```python
from build123d import *

# Parameters (mm, degrees)
F0_W          = 64
F0_H          = 73
F1_DEPTH      = 5.5
F2_DEPTH      = 15.5
F3_W          = 15
F3_H          = 0.5
F4_DEPTH      = 3
F6_W          = 2.5
F6_H          = 15
F7_DEPTH      = 5.501
F8_SIZE       = 2.5
F9_R          = 1.5
F10_R         = 7.5
F11_T1_DEPTH  = 58
F11_T3_DEPTH  = 49
F11_T5_DEPTH  = 2.5
F11_T7_DEPTH  = 15
F11_T10_ANGLE = 90
F11_T12_ANGLE = 90
F11_T14_ANGLE = 90
F11_T16_ANGLE = 90
F11_T21_DEPTH = 5.0870857546
F11_T25_DEPTH = 17.5870857546
F11_T32_DEPTH = 5.0870857546
F11_T36_DEPTH = 17.5870857546
F11_T43_DEPTH = 17.5870857546
F11_T47_DEPTH = 5.0870857546
F11_T54_DEPTH = 5.0870857546
F11_T58_DEPTH = 17.5870857546
F12_SIZE2     = 0.5773502692
F12_SIZE      = 1


# Not quite as in the source:
# - a fillet or chamfer that OpenCascade refuses, or shapes differently, is made with other operations: its cross-section is extruded or revolved along the edge and cut away or added


with BuildPart() as f1:
    # F0 (on Top) → F1 (new body)
    with BuildSketch(Plane.XY):
        Rectangle(F0_W, F0_H)
        Polygon((-22.5, 7.5), (-22.5, 30), (22.5, 30), (22.5, 7.5), (25.5, 7.5), (25.5, -7.5), (22.5, -7.5), (22.5, -30), (-22.5, -30), (-22.5, -7.5), (-25.5, -7.5), (-25.5, 7.5), align=None, mode=Mode.SUBTRACT)
        Polygon((22.5, 30), (-22.5, 30), (-22.5, 7.5), (-25.5, 7.5), (-25.5, -7.5), (-22.5, -7.5), (-22.5, -30), (22.5, -30), (22.5, -7.5), (25.5, -7.5), (25.5, 7.5), (22.5, 7.5), align=None)
    extrude(amount=-F1_DEPTH)

    # F0 (on Top) → F2 (join)
    with BuildSketch(Plane.XY):
        Rectangle(F0_W, F0_H)
        Polygon((-22.5, 7.5), (-22.5, 30), (22.5, 30), (22.5, 7.5), (25.5, 7.5), (25.5, -7.5), (22.5, -7.5), (22.5, -30), (-22.5, -30), (-22.5, -7.5), (-25.5, -7.5), (-25.5, 7.5), align=None, mode=Mode.SUBTRACT)
    extrude(amount=F2_DEPTH)

    # F3 (on face) → F4 (join, through all)
    with BuildSketch(Plane.YZ.offset(-25.5)):
        with Locations((0, 15.25)):
            Rectangle(F3_W, F3_H)
    extrude(amount=F4_DEPTH)

    # F5: F1 across plane


with BuildPart() as f1_1:
    add(f1.part)
    add(f1.part.mirror(Plane.YZ))

    # F6 (on face) → F7 (cut, through all)
    with BuildSketch(Plane.XY):
        with Locations((-17.75, 20.5)):
            Rectangle(F6_W, F6_H)
    extrude(amount=-F7_DEPTH, mode=Mode.SUBTRACT)

    # F8
    f8_edges = [f1_1.edges().sort_by_distance(p)[0] for p in [
        (-22.5, -7.5, 7.5),
        (-22.5, 7.5, 7.5),
        (22.5, 7.5, 7.5),
        (22.5, -7.5, 7.5),
    ]]
    chamfer(f8_edges, length=F8_SIZE)

    # F9
    f9_edges = [f1_1.edges().sort_by_distance(p)[0] for p in [
        (-22.5, 30, 7.75),
        (-22.5, -30, 7.75),
        (22.5, 30, 7.75),
        (22.5, -30, 7.75),
    ]]
    fillet(f9_edges, radius=F9_R)

    # F10
    f10_edges = [f1_1.edges().sort_by_distance(p)[0] for p in [
        (-32, -36.5, 5),
        (32, -36.5, 5),
        (-32, 36.5, 5),
        (32, 36.5, 5),
    ]]
    fillet(f10_edges, radius=F10_R)

    # F11: chamfer of 1 x 0.5773502692 on 12 edges, made by hand

    # F11_s2 → F11_t1 (cut)
    with BuildSketch(Plane.XZ.offset(-29)):
        Polygon((32, -4.5), (31.4226497308, -5.5), (32, -5.5), align=None)
        Polygon((-32, -4.5), (-31.4226497308, -5.5), (-32, -5.5), align=None)
    extrude(amount=F11_T1_DEPTH, mode=Mode.SUBTRACT)

    # F11_s4 → F11_t3 (cut)
    with BuildSketch(Plane.YZ.offset(-24.5)):
        Polygon((-36.5, -4.5), (-35.9226497308, -5.5), (-36.5, -5.5), align=None)
        Polygon((36.5, -4.5), (35.9226497308, -5.5), (36.5, -5.5), align=None)
    extrude(amount=F11_T3_DEPTH, mode=Mode.SUBTRACT)

    # F11_s6 → F11_t5 (cut)
    with BuildSketch(Plane.YZ.offset(-19)):
        Polygon((28.5773502692, -5.5), (28, -4.5), (28, -5.5), align=None)
        Polygon((12.4226497308, -5.5), (13, -4.5), (13, -5.5), align=None)
    extrude(amount=F11_T5_DEPTH, mode=Mode.SUBTRACT)

    # F11_s8 → F11_t7 (cut)
    with BuildSketch(Plane.XZ.offset(-28)):
        Polygon((-19.5773502692, -5.5), (-19, -4.5), (-19, -5.5), align=None)
        Polygon((-15.9226497308, -5.5), (-16.5, -4.5), (-16.5, -5.5), align=None)
    extrude(amount=F11_T7_DEPTH, mode=Mode.SUBTRACT)

    # F11_s9 → F11_t10 (revolve, cut)
    with BuildSketch(Plane.XZ.offset(29)):
        Polygon((32, -4.5), (31.4226497308, -5.5), (32, -5.5), align=None)
    revolve(axis=Axis((24.5, -29, -5.5), (0, 0, -1)), revolution_arc=F11_T10_ANGLE, mode=Mode.SUBTRACT)

    # F11_s11 → F11_t12 (revolve, cut)
    with BuildSketch(Plane.XZ.offset(-29)):
        Polygon((32, -4.5), (31.4226497308, -5.5), (32, -5.5), align=None)
    revolve(axis=Axis((24.5, 29, -5.5), (0, 0, 1)), revolution_arc=F11_T12_ANGLE, mode=Mode.SUBTRACT)

    # F11_s13 → F11_t14 (revolve, cut)
    with BuildSketch(Plane.XZ.offset(29)):
        Polygon((-32, -4.5), (-31.4226497308, -5.5), (-32, -5.5), align=None)
    revolve(axis=Axis((-24.5, -29, -5.5), (0, 0, 1)), revolution_arc=F11_T14_ANGLE, mode=Mode.SUBTRACT)

    # F11_s15 → F11_t16 (revolve, cut)
    with BuildSketch(Plane.YZ.offset(-24.5)):
        Polygon((36.5, -4.5), (35.9226497308, -5.5), (36.5, -5.5), align=None)
    revolve(axis=Axis((-24.5, 29, -5.5), (0, 0, 1)), revolution_arc=F11_T16_ANGLE, mode=Mode.SUBTRACT)


with BuildPart() as f11_tool19:
    # F11_s20 → F11_t21 (new body)
    with BuildSketch(Plane.YZ.offset(-13.9129142454)):
        Polygon((28.5773502692, -5.5), (28, -4.5), (28, -5.5), align=None)
    extrude(amount=-F11_T21_DEPTH)

    split(bisect_by=Plane.YZ.offset(-16.5), keep=Keep.TOP)


with BuildPart() as f11_tool23:
    # F11_s24 → F11_t25 (new body)
    with BuildSketch(Plane.XZ.offset(-13)):
        Polygon((-15.9226497308, -5.5), (-16.5, -4.5), (-16.5, -5.5), align=None)
    extrude(amount=-F11_T25_DEPTH)

    split(bisect_by=Plane.XZ.offset(-28), keep=Keep.BOTTOM)


with BuildPart() as f11_tool19_1:
    add(f11_tool19.part)

    # F11_t27: intersect F11_tool23
    add(f11_tool23.part, mode=Mode.INTERSECT)


with BuildPart() as f1_2:
    add(f1_1.part)

    # F11_t17: cut F11_tool19
    add(f11_tool19_1.part, mode=Mode.SUBTRACT)


with BuildPart() as f11_tool30:
    # F11_s31 → F11_t32 (new body)
    with BuildSketch(Plane.YZ.offset(-16.5)):
        Polygon((28.5773502692, -5.5), (28, -4.5), (28, -5.5), align=None)
    extrude(amount=-F11_T32_DEPTH)

    split(bisect_by=Plane.YZ.offset(-19), keep=Keep.BOTTOM)


with BuildPart() as f11_tool34:
    # F11_s35 → F11_t36 (new body)
    with BuildSketch(Plane.XZ.offset(-30.5870857546)):
        Polygon((-19.5773502692, -5.5), (-19, -4.5), (-19, -5.5), align=None)
    extrude(amount=F11_T36_DEPTH)

    split(bisect_by=Plane.XZ.offset(-28), keep=Keep.BOTTOM)


with BuildPart() as f11_tool30_1:
    add(f11_tool30.part)

    # F11_t38: intersect F11_tool34
    add(f11_tool34.part, mode=Mode.INTERSECT)


with BuildPart() as f1_3:
    add(f1_2.part)

    # F11_t28: cut F11_tool30
    add(f11_tool30_1.part, mode=Mode.SUBTRACT)


with BuildPart() as f11_tool41:
    # F11_s42 → F11_t43 (new body)
    with BuildSketch(Plane.XZ.offset(-28)):
        Polygon((-19.5773502692, -5.5), (-19, -4.5), (-19, -5.5), align=None)
    extrude(amount=F11_T43_DEPTH)

    split(bisect_by=Plane.XZ.offset(-13), keep=Keep.TOP)


with BuildPart() as f11_tool45:
    # F11_s46 → F11_t47 (new body)
    with BuildSketch(Plane.YZ.offset(-21.5870857546)):
        Polygon((12.4226497308, -5.5), (13, -4.5), (13, -5.5), align=None)
    extrude(amount=F11_T47_DEPTH)

    split(bisect_by=Plane.YZ.offset(-19), keep=Keep.BOTTOM)


with BuildPart() as f11_tool41_1:
    add(f11_tool41.part)

    # F11_t49: intersect F11_tool45
    add(f11_tool45.part, mode=Mode.INTERSECT)


with BuildPart() as f1_4:
    add(f1_3.part)

    # F11_t39: cut F11_tool41
    add(f11_tool41_1.part, mode=Mode.SUBTRACT)


with BuildPart() as f11_tool52:
    # F11_s53 → F11_t54 (new body)
    with BuildSketch(Plane.YZ.offset(-19)):
        Polygon((12.4226497308, -5.5), (13, -4.5), (13, -5.5), align=None)
    extrude(amount=F11_T54_DEPTH)

    split(bisect_by=Plane.YZ.offset(-16.5), keep=Keep.TOP)


with BuildPart() as f11_tool56:
    # F11_s57 → F11_t58 (new body)
    with BuildSketch(Plane.XZ.offset(-10.4129142454)):
        Polygon((-15.9226497308, -5.5), (-16.5, -4.5), (-16.5, -5.5), align=None)
    extrude(amount=-F11_T58_DEPTH)

    split(bisect_by=Plane.XZ.offset(-13), keep=Keep.TOP)


with BuildPart() as f11_tool52_1:
    add(f11_tool52.part)

    # F11_t60: intersect F11_tool56
    add(f11_tool56.part, mode=Mode.INTERSECT)


with BuildPart() as f1_5:
    add(f1_4.part)

    # F11_t50: cut F11_tool52
    add(f11_tool52_1.part, mode=Mode.SUBTRACT)

    # F12
    f12_edges = [f1_5.edges().sort_by_distance(p)[0] for p in [
        (-29.803301, -34.303301, 15.5),
        (-32, 0, 15.5),
        (0, -36.5, 15.5),
        (29.803301, -34.303301, 15.5),
        (32, 0, 15.5),
        (29.803301, 34.303301, 15.5),
        (0, 36.5, 15.5),
        (-29.803301, 34.303301, 15.5),
    ]]
    chamfer(f12_edges, length=F12_SIZE, length2=F12_SIZE2)


solid = f1_5.part
```
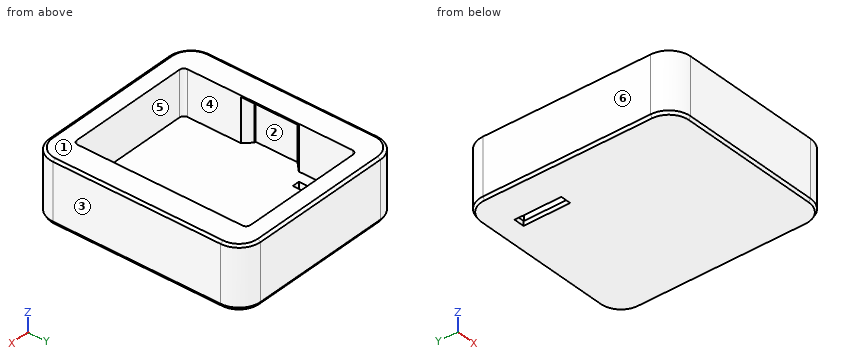
Input: part model. Units: mm. Frame: model coordinates. Face numbers are marked on the shaded views. A direction names the side the tool comes from. Coordinates: 2 decimals unless noted, no trailing zeros. Loops run counter-clockwise (first coordinate to the right, second up) from the corner with the lowest first, then second, coordinate; pieces in that order, holes last. Notation, with made-up numbers: (17.25, -3.5) - (74.25, -3.5) arc R13 ccw to (74.25, 7.5) - close; hole circle Ø2 at (5.25, 10). An arc over 180 degrees is marked (long way). Answer in a Markdown table with one row per item.
(1) Cut plane A-A on z = 11.5. Output: boundary loops of the cut face in (x, y), plus the area to 3 significant figures.
Model answer:
| item | result |
|---|---|
| outline | (-32, -29) arc R7.5 ccw to (-24.5, -36.5) - (24.5, -36.5) arc R7.5 ccw to (32, -29) - (32, 29) arc R7.5 ccw to (24.5, 36.5) - (-24.5, 36.5) arc R7.5 ccw to (-32, 29) - close; hole (-25.5, -7.5) - (-25, -7.5) - (-22.5, -10) - (-22.5, -28.5) arc R1.5 ccw to (-21, -30) - (21, -30) arc R1.5 ccw to (22.5, -28.5) - (22.5, -10) - (25, -7.5) - (25.5, -7.5) - (25.5, 7.5) - (25, 7.5) - (22.5, 10) - (22.5, 28.5) arc R1.5 ccw to (21, 30) - (-21, 30) arc R1.5 ccw to (-22.5, 28.5) - (-22.5, 10) - (-25, 7.5) - (-25.5, 7.5) - close |
| area | 1,820 mm² |
(2) Set-up query: the marked faces 5 and 6. Return all of +Z, -Z, +X, -X, +Y, -Y with unobstructed straight access to the full face (end or side cutting, diameter ignored); none if empty.
Model answer:
| item | result |
|---|---|
| face 5 | +Z |
| face 6 | +Z, -Z, -X, +Y, -Y |
(3) Cut plane B-B on y = -23. Output: boundary loops of the cut face in (x, z), plus the area to 3 significant figures.
Model answer:
| item | result |
|---|---|
| outline | (-32, -4.5) - (-31.42, -5.5) - (31.42, -5.5) - (32, -4.5) - (32, 14.92) - (31, 15.5) - (22.5, 15.5) - (22.5, 0) - (-22.5, 0) - (-22.5, 15.5) - (-31, 15.5) - (-32, 14.92) - close |
| area | 645 mm² |
(4) Material intervals for L1, parallel to X at y = -2, z = 13.5; L2, parallel to X at y = 20.5, z = 3; L3, parallel to Y at x = 15.5, z = 8.25, sorted ascending. Write a range as from..to.
Model answer:
| item | result |
|---|---|
| L1 | x = -32..-25.5, 25.5..32 |
| L2 | x = -32..-22.5, 22.5..32 |
| L3 | y = -36.5..-30, 30..36.5 |
(5) Cut plane D-D on z = -2.5. Output: boundary loops of the cut face in (x, y).
Model answer:
| item | result |
|---|---|
| outline | (-32, -29) arc R7.5 ccw to (-24.5, -36.5) - (24.5, -36.5) arc R7.5 ccw to (32, -29) - (32, 29) arc R7.5 ccw to (24.5, 36.5) - (-24.5, 36.5) arc R7.5 ccw to (-32, 29) - close; hole (-19, 13) - (-16.5, 13) - (-16.5, 28) - (-19, 28) - close |
(6) Mould query, pull axis X, two halves, no side actions, for the marked faces 1, 2, 3 and 4. Classes: pulls with the +X half, pulls with the -X half, needs draft (parallel to the pull), parting line crosses it, or undercut.
Model answer:
| item | result |
|---|---|
| face 1 | needs draft |
| face 2 | undercut |
| face 3 | pulls with the +X half |
| face 4 | undercut |
(7) Pin query (flat end, axial travel): P1, Ø0.6, axis at x = -25, z = 6, coming from the +Y side. Return the tip coordinate at first contact, or that it passes through.
Model answer:
| item | result |
|---|---|
| P1 | stops at y = 36.5 |
(8) Cut plane C-C on x = 9. Output: boundary loops of the cut face in (y, z), plus the area to 3 significant figures.
Model answer:
| item | result |
|---|---|
| outline | (-36.5, -4.5) - (-35.92, -5.5) - (35.92, -5.5) - (36.5, -4.5) - (36.5, 14.92) - (35.5, 15.5) - (30, 15.5) - (30, 0) - (-30, 0) - (-30, 15.5) - (-35.5, 15.5) - (-36.5, 14.92) - close |
| area | 602 mm² |
